Drawing for the job (mm, zero at the part's lowest x, y, z). Coordinates: 2 decimals unless noted, no trailing zeros. Order: outer loops, then holes, each group sorted by start corner. A loop starts at its lowest first (then second) coordinate and runs counter-clockwise, first axis right, second up.
1) Cut at B-B (z = 10). List the corners of the cut face in (x, y).
2) Cut at A-A (x = 10). List the corners of the cut face in (y, z).
3) Wall check: L1, parallel to X at y = 3.75, z = 34; L2, parallel to Z at x = 10, y = 2.5; L3, parallel to Z at x = 100, y = 4.75. Give the ranges that are in metal, low to high.
4) Pin check, flat tips, straight feed: pin 1 Ø2 at (x, y) = (83, 3) entering from +Z; pin 2 Ø1 at (y, z) = (4, 63) entering from +X; pin 3 Ø3 at (x, y) = (71.5, 2) entering from -Z. Stop position of each tip, or through.
5) Cut at C-C (y = 4.5). List the corners of the cut face in (x, z) (1 decimal).
6) Cut at D-D (x = 53.5). List the corners of the cut face in (y, z), and give its area (3 significant figures).
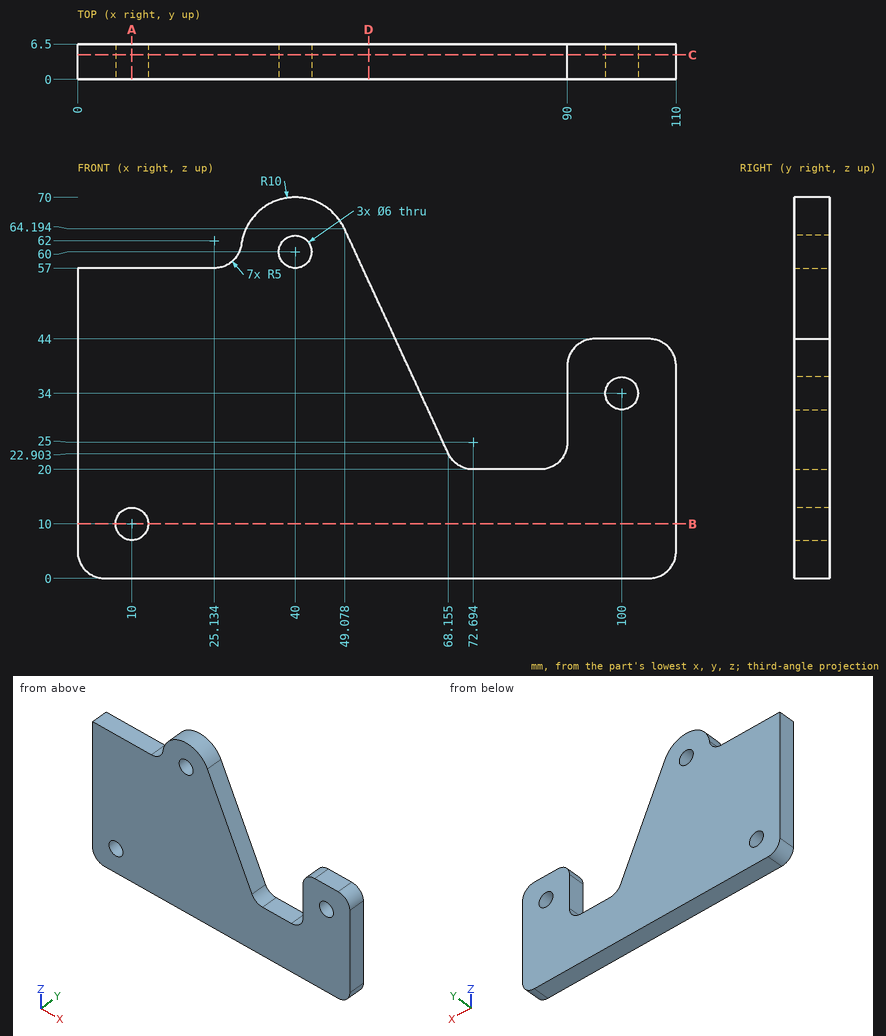
Geometry check:
1. outline: (0, 0) - (7, 0) - (7, 6.5) - (0, 6.5) - close; (13, 0) - (110, 0) - (110, 6.5) - (13, 6.5) - close
2. outline: (0, 0) - (6.5, 0) - (6.5, 7) - (0, 7) - close; (0, 13) - (6.5, 13) - (6.5, 57) - (0, 57) - close
3. L1: x = 0 to 63.03, 90 to 97, 103 to 110
3. L2: z = 0 to 7, 13 to 57
3. L3: z = 0 to 31, 37 to 44
4. pin 1: stops at z = 20
4. pin 2: stops at x = 49.86
4. pin 3: stops at z = 0
5. outline: (0, 5) arc R5 ccw to (5, 0) - (105, 0) arc R5 ccw to (110, 5) - (110, 39) arc R5 ccw to (105, 44) - (95, 44) arc R5 ccw to (90, 39) - (90, 25) arc R5 cw to (85, 20) - (72.7, 20) arc R5 cw to (68.2, 22.9) - (49.1, 64.2) arc R10 ccw to (30.1, 61.3) arc R5 cw to (25.1, 57) - (0, 57) - close; hole circle Ø6 at (10, 10); hole circle Ø6 at (40, 60); hole circle Ø6 at (100, 34)
6. outline: (0, 0) - (6.5, 0) - (6.5, 54.62) - (0, 54.62) - close
6. area: 355 mm2
